Work out the finished part from the listing and answer in its coordinate system (mm). A direction names the side the tool comes from. Round coordinates to 2 decimals unless told otherwise and drop trailing zeros. Write each loop counter-clockwise with the first axis right and the second up, starting at its lowest first coordinate (ties: lowest second). Pieces come first, ordered by that corner, then holes. Notation, with made-up numbers: M 88,48.5 L 118,48.5 A16 cw 118,52.5 Z; hole C -37,88.5 d11. An arc over 180 degrees is marked long. Answer in a Markdown table with one row per item.
Autodesk Inventor part; units mm, degrees
ref_plane "YZ Plane" through (0, 0, 0) normal (1, 0, 0) x (0, 1, 0)
ref_plane "XZ Plane" through (0, 0, 0) normal (0, 1, 0) x (-1, 0, 0)
ref_plane "XY Plane" through (0, 0, 0) normal (0, 0, 1) x (1, 0, 0)
sketch "Sketch1" plane through (0, 0, 0) normal (0, 1, 0) x (-1, 0, 0)
  circle A0 centre (0, 0) radius 2.8
  dimension "d0" = 5.6
extrude "Extrusion1" add sketch "Sketch1" along normal blind 9
chamfer "Chamfer1" distance 1 angle 45 1 edges at (2.8, 9, 0)
sketch "Sketch3" plane through (0, 0, 0) normal (1, 0, 0) x (0, 1, 0)
  line L0 (0, -2.8) -> (8, -2.8)
  line L1 (3.2, -2.8) -> (0, -2.8)
  line L2 (0, -2.8) -> (0, -3.3)
  line L3 (0, -3.3) -> (3.2, -3.3)
  line L4 (3.2, -3.3) -> (3.2, -2.8)
  line L5 (0, 2.8) -> (0, -2.8)
  line L6 (-1.8, 0) -> (10.8, 0)
  point P0 (0, 0)
  dimension "d9" = 3.2
  dimension "d11" = 0.5
revolve "Revolution1" add sketch "Sketch3" angle 360 about axis through (0, -10, 0) along (0, 1, 0)
properties part number "Knopf"
1. The part is cut by section C-C (y = 2.25). Determine the outline of the cut face in (x, z), plus the area to 3 significant figures.
Calculated:
| item | result |
|---|---|
| outline | C 0,0 d6.6 |
| area | 34.2 mm² |
2. The part is cut by section A-A (x = 0). Determine the outline of the cut face in (y, z).
Calculated:
| item | result |
|---|---|
| outline | M 0,-3.3 L 3.2,-3.3 L 3.2,-2.8 L 8,-2.8 L 9,-1.8 L 9,1.8 L 8,2.8 L 3.2,2.8 L 3.2,3.3 L 0,3.3 Z |
3. A tool of negligible diameter and unlimited length cuts with its end or side. For faces 1 (the flat face through (0, 9, 0)), 2 (the cylindrical face through (2.8, 5.6, -0.1)), from which of +Z, -Z, +X, -X, +Y, -Y can it reach the whole face along a straight path? Write none if from no direction.
Calculated:
| item | result |
|---|---|
| face 1 | +Z, -Z, +X, -X, +Y |
| face 2 | +Y |
4. Given pin 1 (1.5 mm diameter, centred on x = -1.5, y = 5.5, fed in from +Z); pin 2 (1 mm diameter, centred on y = 6.5, z = 1.5, fed in from -X); pin 3 (1 mm diameter, centred on y = 1, z = 1.5, fed in from -X), each flat-ended and moving along its own axis, determine where each tip first touches the part or whether it passes through.
Calculated:
| item | result |
|---|---|
| pin 1 | stops at z = 2.7 |
| pin 2 | stops at x = -2.62 |
| pin 3 | stops at x = -3.14 |
5. Consider line 1 along X through (y, z) = (3.25, 0); line 2 along Y through (x, z) = (-2.75, -1.25); line 3 along X through (y, z) = (7.25, -1.5). Determine where each line is inside the solid, lowest interval first. Write a range as from..to.
Calculated:
| item | result |
|---|---|
| line 1 | x = -2.8..2.8 |
| line 2 | y = 0..3.2 |
| line 3 | x = -2.36..2.36 |
6. The part is cut by section B-B (z = 0). Determine the outline of the cut face in (x, y), plus the area to 3 significant figures.
Calculated:
| item | result |
|---|---|
| outline | M -3.3,0 L 3.3,0 L 3.3,3.2 L 2.8,3.2 L 2.8,8 L 1.8,9 L -1.8,9 L -2.8,8 L -2.8,3.2 L -3.3,3.2 Z |
| area | 52.6 mm² |
7. The part is cut by section D-D (y = 4). Determine the outline of the cut face in (x, z), plus the area to 3 significant figures.
Calculated:
| item | result |
|---|---|
| outline | C 0,0 d5.6 |
| area | 24.6 mm² |
